from build123d import *

# Parameters (mm, degrees)
POCKET_DEPTH = 5
CHAMFER_SIZE = 0.5


with BuildPart() as part:
    # Sketch → Revolution (revolve)
    with BuildSketch(Plane.XZ):
        Polygon((-2, -10), (-3.45, -10), (-3.45, 0), (-5.1, 0), (-5.1, 25), (-2, 25), align=None)
    revolve(axis=Axis((0, 0, 0), (0, 0, 1)))

    # Sketch001 (on Face5 of Revolution) → Pocket (cut)
    with BuildSketch(Plane(origin=(0, 0, 25), x_dir=(-1, 0, 0), z_dir=(0, 0, 1))):
        Polygon((2.092895, -3.625), (4.185789, 0), (2.092895, 3.625), (-2.092895, 3.625), (-4.185789, 0), (-2.092895, -3.625), align=None)
    extrude(amount=-POCKET_DEPTH, mode=Mode.SUBTRACT)

    # Chamfer
    chamfer_edges = [part.edges().sort_by_distance(p)[0] for p in [
        (3.45, 0, -10),
        (5.1, 0, 0),
        (5.1, 0, 25),
    ]]
    chamfer(chamfer_edges, length=CHAMFER_SIZE)


solid = part.part
Model file for the job. Use its own axes, mm. A direction names the side the tool comes from. Round coordinates to 2 decimals unless told otherwise and drop trailing zeros. Order: outer loops, then holes, each group sorted by start corner. A loop starts at its lowest first (then second) coordinate and runs counter-clockwise, first axis right, second up.
(1) Drill centre lines: line 1 (Y direction, x = 0, z = 12.5); line 2 (X direction, y = 0, z = -3.25). Where is each one in solid material? Low to high.
(2) 3-axis set-ups, long thin cutter, end or side, ignore diameter. For faces 1 (the face through (2, -1, 20)), 2 (the face through (0, 2, 5)), 3 (the face through (0.45, -3.42, -4.68)): which of +Z, -Z, +X, -X, +Y, -Y reach the whole face in a straight line?
(3) Pull direction Y, two halves, no side cores. Call faces 4 (the face through (2, 1, -10)), 5 (the face through (-2.4, 4.5, 12.7)), 6 (the face through (-3.154, -1.787, 22.535)): released by +Y, released by -Y, zero draft, split by the parting line, or undercut.
(4) Pin check, flat tips, straight feed: pin 1 (1 mm diameter, centred on y = -2.5, z = 3.5, fed in from +X); pin 2 (3 mm diameter, centred on x = -3.5, z = -5, fed in from -Y); pin 3 (2 mm diameter, centred on x = 0.5, y = -4, fed in from -Z). Stop position of each tip, or through.
(5) Band-saw the part on B-B (z = 19.5). List the corners of the cut face in (x, y), then the cut area to 3 significant figures.
(6) Band-saw the part on A-A (x = 0). List the corners of the cut face in (y, z) (3 decimals).
Verdict:
1. line 1: y = -5.1 to -2, 2 to 5.1
1. line 2: x = -3.45 to -2, 2 to 3.45
2. face 1: +Z
2. face 2: +Z, -Z
2. face 3: -Z
3. face 4: zero draft
3. face 5: split by the parting line
3. face 6: undercut
4. pin 1: stops at x = 4.69
4. pin 2: stops at y = -2.81
4. pin 3: stops at z = -9.92
5. outline: circle Ø10.2 at (0, 0); hole circle Ø4 at (0, 0)
5. area: 69.1 mm2
6. outline: (-5.1, 0.5) - (-4.6, 0) - (-3.45, 0) - (-3.45, -9.5) - (-2.95, -10) - (-2, -10) - (-2, 20) - (-3.625, 20) - (-3.625, 25) - (-4.6, 25) - (-5.1, 24.5) - close; (2, -10) - (2.95, -10) - (3.45, -9.5) - (3.45, 0) - (4.6, 0) - (5.1, 0.5) - (5.1, 24.5) - (4.6, 25) - (3.625, 25) - (3.625, 20) - (2, 20) - close
